Check sheet for the modelled part. Datum: model origin and axes. Units: mm. Face numbers are marked on the shaded views. A direction names the side the tool comes from. Round coordinates to 2 decimals unless told otherwise and drop trailing zeros. Order: outer loops, then holes, each group sorted by start corner. A loop starts at its lowest first (then second) coordinate and runs counter-clockwise, first axis right, second up. Notation, with made-up numbers: (5, 9) -> (22, 9) arc R20 cw to (22, 48) -> close; hole circle Ø7 at (71, 23). An arc over 180 degrees is marked (long way). Answer in a Markdown table with one row per item.
from build123d import *

# Parameters (mm, degrees)
ESQUISSE1_W             = 6.9
ESQUISSE1_H             = 6.9
BOSS_EXTRU_1_DEPTH      = 1.5
ESQUISSE2_R             = 3.4
ENL_V_MAT_EXTRU_7_DEPTH = 1
ENL_V_MAT_EXTRU_8_DEPTH = 1
ESQUISSE4_W             = 6.9
ESQUISSE4_H             = 2.359638985
ENL_V_MAT_EXTRU_9_DEPTH = 0.5
CHANFREIN1_SIZE         = 1
CONG_1_R                = 0.5


with BuildPart() as part:
    # Esquisse1 → Boss.-Extru.1 (new body)
    with BuildSketch(Plane.XY):
        with Locations((3.45, 3.45)):
            Rectangle(ESQUISSE1_W, ESQUISSE1_H)
    extrude(amount=BOSS_EXTRU_1_DEPTH)

    # Esquisse2 → Enlèv. mat.-Extru.7 (cut)
    with BuildSketch(Plane.XY.offset(1.5)):
        with Locations((3.45, 3.45)):
            Circle(ESQUISSE2_R)
    extrude(amount=-ENL_V_MAT_EXTRU_7_DEPTH, mode=Mode.SUBTRACT)

    # Esquisse3 → Enlèv. mat.-Extru.8 (cut)
    with BuildSketch(Plane.XY.offset(1.5)):
        Polygon((0, 4.540361015), (2.36, 4.540361015), (2.36, 6.9), (4.54, 6.9), (4.54, 4.540361015), (6.9, 4.540361015), (6.9, 2.359638985), (4.54, 2.359638985), (4.54, 0), (2.36, 0), (2.36, 2.359638985), (0, 2.359638985), align=None)
    extrude(amount=-ENL_V_MAT_EXTRU_8_DEPTH, mode=Mode.SUBTRACT)

    # Esquisse4 → Enlèv. mat.-Extru.9 (cut)
    with BuildSketch(Plane.XY.offset(1.5)):
        with Locations((3.45, 1.179819493)):
            Rectangle(ESQUISSE4_W, ESQUISSE4_H)
    extrude(amount=-ENL_V_MAT_EXTRU_9_DEPTH, mode=Mode.SUBTRACT)

    # Chanfrein1
    chanfrein1_edges = [part.edges().sort_by_distance(p)[0] for p in [
        (6.9, 0, 0.5),
        (0, 0, 0.5),
    ]]
    chamfer(chanfrein1_edges, length=CHANFREIN1_SIZE)

    # Congé1
    cong_1_edges = [part.edges().sort_by_distance(p)[0] for p in [
        (0, 6.9, 0.75),
        (6.9, 6.9, 0.75),
    ]]
    fillet(cong_1_edges, radius=CONG_1_R)


solid = part.part
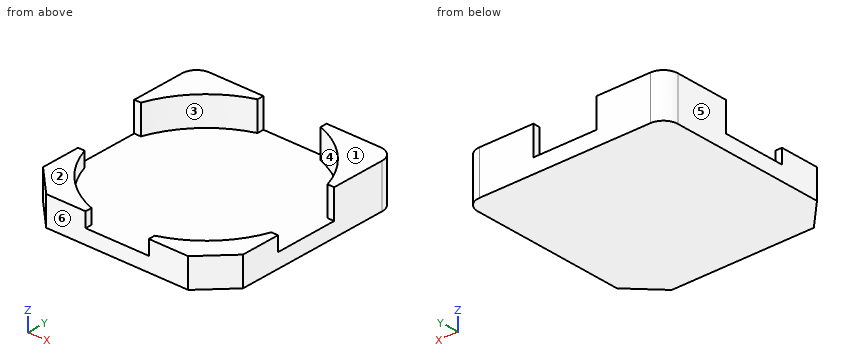
Item 1: Mould release check, pull along Y, two halves, no side actions. Record for the marked faces 4, 5 and 6: pulls with the +Y half, pulls with the -Y half, needs draft (parallel to the pull), parting line crosses it, or undercut.
Result sheet:
| item | result |
|---|---|
| face 4 | undercut |
| face 5 | needs draft |
| face 6 | pulls with the -Y half |
Item 2: Cross-section at C-C (x = 6). Record the boundary of the cut face in (y, z).
Result sheet:
| item | result |
|---|---|
| outline | (0.1, 0) -> (6.9, 0) -> (6.9, 1.5) -> (5.7, 1.5) -> (5.7, 0.5) -> (1.2, 0.5) -> (1.2, 1) -> (0.1, 1) -> close |
Item 3: Cross-section at B-B (z = 0.35). Record the boundary of the cut face in (x, y), and give its area (3 significant figures).
Result sheet:
| item | result |
|---|---|
| outline | (0, 1) -> (1, 0) -> (5.9, 0) -> (6.9, 1) -> (6.9, 6.4) arc R0.5 ccw to (6.4, 6.9) -> (0.5, 6.9) arc R0.5 ccw to (0, 6.4) -> close |
| area | 46.5 mm^2 |
Item 4: Cross-section at D-D (y = 2.5). Record the boundary of the cut face in (x, z), and give its area (3 significant figures).
Result sheet:
| item | result |
|---|---|
| outline | (0, 0) -> (6.9, 0) -> (6.9, 0.5) -> (0, 0.5) -> close |
| area | 3.45 mm^2 |
Item 5: Depth check by flat-ended pin: P1, Ø1.5, axis at x = 6, y = 1.5, coming from the -Z side; P2, Ø1.9, axis at x = 1, y = 1, coming from the +Z side; P3, Ø2, axis at x = 5, y = 4.5, coming from the +Z side. Enter the tip coordinate at first touch or a pass-through.
Result sheet:
| item | result |
|---|---|
| P1 | stops at z = 0 |
| P2 | stops at z = 1 |
| P3 | stops at z = 0.5 |
Item 6: Cross-section at A-A (z = 1.2). Record the boundary of the cut face in (x, y), and give its area (3 significant figures).
Result sheet:
| item | result |
|---|---|
| outline | (0, 4.54) -> (0.23, 4.54) arc R3.4 cw to (2.36, 6.67) -> (2.36, 6.9) -> (0.5, 6.9) arc R0.5 ccw to (0, 6.4) -> close; (4.54, 6.67) arc R3.4 cw to (6.67, 4.54) -> (6.9, 4.54) -> (6.9, 6.4) arc R0.5 ccw to (6.4, 6.9) -> (4.54, 6.9) -> close |
| area | 5.06 mm^2 |
Item 7: Scan lines: line 1 (Z direction, x = 4.25, y = 2.75); line 2 (Z direction, x = 6.5, y = 1.75); line 3 (X direction, y = 5.75, z = 1). Record each from-to range of solid material in increasing order. Write a range as [from, to].
Result sheet:
| item | result |
|---|---|
| line 1 | z = [0, 0.5] |
| line 2 | z = [0, 1] |
| line 3 | x = [0, 0.95], [5.95, 6.9] |
Item 8: Set-up check for the marked faces 1, 2 and 3: record each of +Z, -Z, +X, -X, +Y, -Y from which the full face is reachable in a straight line by a thin tool's end or side.
Result sheet:
| item | result |
|---|---|
| face 1 | +Z, +X, -X, +Y, -Y |
| face 2 | +Z, +X, -X, -Y |
| face 3 | +Z |
